Check sheet for the drawn part. Datum: minimum x, y, z corner. Units: mm. Round coordinates to 2 decimals unless told otherwise and drop trailing zeros. Loops run counter-clockwise (first coordinate to the right, second up) from the corner with the lowest first, then second, coordinate; pieces in that order, holes last. Notation, with made-up numbers: (29, 49) -> (64, 49) arc R24 ccw to (64, 69) -> close; hole circle Ø1 at (45, 34.25). An arc over 180 degrees is marked (long way). Return JSON: item names as keys, results as strings.
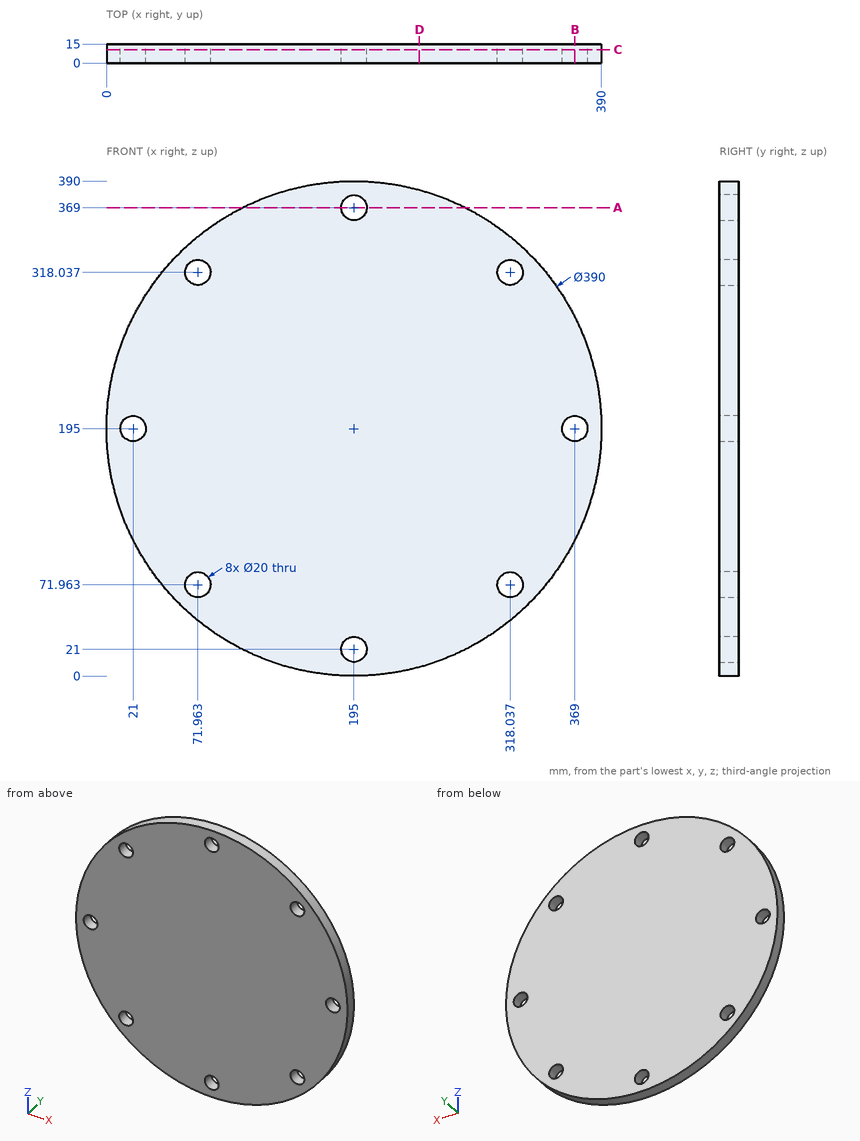
Q1. Section check B-B (x = 369). Record the boundary of the cut face in (y, z).
Results list:
{"outline": "(0, 106.97) -> (15, 106.97) -> (15, 185) -> (0, 185) -> close; (0, 205) -> (15, 205) -> (15, 283.03) -> (0, 283.03) -> close"}
Q2. Section check C-C (y = 10.5). Count the separate pieces of the cut face and the enclosed holes in it, then the cut area to 3 significant figures.
Results list:
{"separate pieces": "1", "enclosed holes": "8", "area": "117,000 mm^2"}
Q3. Section check D-D (x = 246.5). Record the boundary of the cut face in (y, z).
Results list:
{"outline": "(0, 6.92) -> (15, 6.92) -> (15, 383.08) -> (0, 383.08) -> close"}
Q4. Go/stop test with flat-tipped pins: pin 1 (4 mm diameter, centred on x = 123.5, y = 13, fed in from -Z) (1 decimal); pin 2 (4 mm diameter, centred on x = 299.5, y = 3.5, fed in from +Z); pin 3 (4 mm diameter, centred on x = 155, y = 2, fed in from +Z). Record where each tip stops, or that it passes through.
Results list:
{"pin 1": "z = 12.8", "pin 2": "z = 360.89", "pin 3": "z = 386.26"}
Q5. Material ranges on line 1 (X direction, y = 9.75, z = 195); line 2 (Z direction, x = 198.5, y = 11); line 3 (X direction, y = 2.75, z = 323) (1 decimal), recorded low to high.
Results list:
{"line 1": "0 to 11, 31 to 359, 379 to 390", "line 2": "0.03 to 11.63, 30.37 to 359.63, 378.37 to 389.97", "line 3": "47.9 to 63.3, 80.6 to 309.4, 326.7 to 342.1"}
Q6. Section check A-A (z = 369). Record the boundary of the cut face in (x, y).
Results list:
{"outline": "(106.97, 0) -> (185, 0) -> (185, 15) -> (106.97, 15) -> close; (205, 0) -> (283.03, 0) -> (283.03, 15) -> (205, 15) -> close"}
